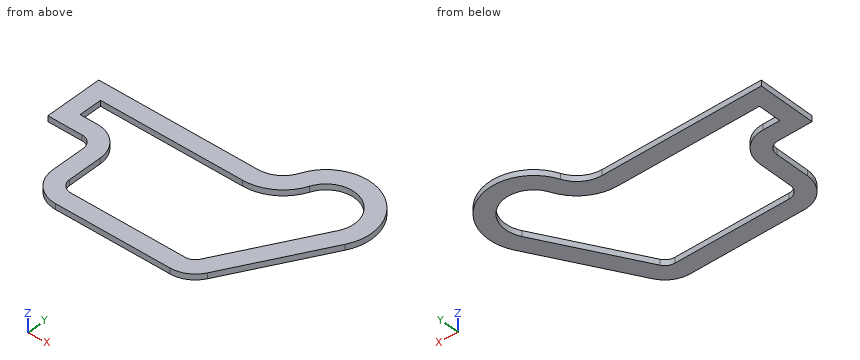
from build123d import *

# Parameters (mm, degrees)
BOSS_EXTRUDE1_DEPTH = 5
SHELL1_T            = -15


with BuildPart() as part:
    # Sketch3 → Boss-Extrude1 (new body)
    with BuildSketch(Plane.XY):
        with BuildLine():
            Line((140, 115), (0, 115))
            Line((0, 115), (0, 65))
            Line((0, 65), (30, 65))
            ThreePointArc((30, 65), (37.071067812, 62.071067812), (40, 55))
            Line((40, 55), (40, 25))
            ThreePointArc((40, 25), (47.32233047, 7.32233047), (65, 0))
            Line((65, 0), (165.538941775, 0))
            ThreePointArc((165.538941775, 0), (178.05666204, 3.359605379), (187.210014279, 12.535465651))
            Line((187.210014279, 12.535465651), (234.673716006, 95.056745042))
            ThreePointArc((234.673716006, 95.056745042), (217.699703722, 150.870886358), (163.076923077, 130.384615385))
            ThreePointArc((163.076923077, 130.384615385), (153.867504906, 119.198742642), (140, 115))
        make_face()
    extrude(amount=BOSS_EXTRUDE1_DEPTH)

    # Shell1
    shell1_openings = [part.faces().sort_by_distance(p)[0] for p in [
        (98.657145907, 64.238067092, 5),
        (98.657145907, 64.238067092, 0),
    ]]
    offset(amount=SHELL1_T, openings=shell1_openings, kind=Kind.INTERSECTION)


solid = part.part
Check sheet for the modelled part. Datum: model origin and axes. Units: mm. Give positions to 0.01 mm unless a question says otherwise; leave off trailing zeros. Order: outer loops, then holes, each group sorted by start corner. A loop starts at its lowest first (then second) coordinate and runs counter-clockwise, first axis right, second up. Notation, with made-up numbers: M 5.5,71.25 L 31.5,71.25 A16 ccw 31.5,95.25 Z; hole C 41,-22 d11. An arc over 180 degrees is marked long. Answer as CSV lines item,"result". Start each with the question number.
Item 1: Cross-section at C-C on y = 106.5. Enter the section's corners in (x, z), plus the area to 3 significant figures.
Item 2: Cross-section at B-B on x = 67.5. Enter the section's corners in (y, z).
Item 3: Cross-section at A-A on z = 2.8. Enter the section's corners in (x, y).
Item 4: Thickness scan on line 1 (Y direction, x = 99, z = 2.45); line 2 (Y direction, x = 28, z = 2.45); line 3 (X direction, y = 28.5, z = 3.85). Record the ranges inside material, lowest first. Write a range as [from, to].
Item 5: Gauge pin test, flat ends, axial feed: P1, Ø2, axis at y = 112.5, z = 3.5, coming from the +X side; P2, Ø1.5, axis at x = 19, z = 3.5, coming from the +Y side; P3, Ø1, axis at y = 57.5, z = 4.5, coming from the +X side. Record the tip position at first contact, or that the pin passes through.
Established:
1,outline,"M 0,0 L 161.86,0 L 161.86,5 L 0,5 Z; M 223.51,0 L 239.09,0 L 239.09,5 L 223.51,5 Z"
1,area,"887 mm^2"
2,outline,"M 0,0 L 15,0 L 15,5 L 0,5 Z; M 100,0 L 115,0 L 115,5 L 100,5 Z"
3,outline,"M 0,65 L 30,65 A10 cw 40,55 L 40,25 A25 ccw 65,0 L 165.54,0 A25 ccw 187.21,12.54 L 234.67,95.06 A40 ccw long 163.08,130.38 A25 cw 140,115 L 0,115 Z; hole M 15,80 L 30,80 A25 cw 55,55 L 55,25 A10 ccw 65,15 L 165.54,15 A10 ccw 174.21,20.01 L 221.67,102.54 A25 ccw long 176.92,124.62 A40 cw 140,100 L 15,100 Z"
4,line 1,"y = [0, 15], [100, 115]"
4,line 2,"y = [65, 80], [100, 115]"
4,line 3,"x = [40, 55], [179.09, 196.39]"
5,P1,"stops at x = 239.97"
5,P2,"stops at y = 115"
5,P3,"stops at x = 213.36"
